from build123d import *

# Parameters (mm, degrees)
SKETCH1_R           = 2.55
SKETCH1_R_2         = 2.5
SKETCH1_R_3         = 10
BOSS_EXTRUDE1_DEPTH = 6.35


with BuildPart() as part:
    # Sketch1 → Boss-Extrude1 (new body)
    with BuildSketch(Plane(origin=(0, 0, 0), x_dir=(1, 0, 0), z_dir=(0, 1, 0))):
        with BuildLine():
            ThreePointArc((-155, 42.5), (-197.5, 0), (-155, -42.5))
            Line((-155, -42.5), (0, -42.5))
            ThreePointArc((0, -42.5), (42.200640469, -5.0354686), (10, 41.306779105))
            Line((10, 41.306779105), (10, 52.5))
            ThreePointArc((10, 52.5), (0, 62.5), (-10, 52.5))
            Line((-10, 52.5), (-10, 42.5))
            Line((-10, 42.5), (-155, 42.5))
        make_face()
        with BuildLine():
            ThreePointArc((-115, 2.55), (-112.45, 0), (-115, -2.55))
            Line((-115, -2.55), (-130, -2.55))
            ThreePointArc((-130, -2.55), (-132.55, 0), (-130, 2.55))
            Line((-130, 2.55), (-115, 2.55))
        make_face(mode=Mode.SUBTRACT)
        with Locations(Location((-155, -37.5, 0), (0, 0, 270))):
            Circle(SKETCH1_R, mode=Mode.SUBTRACT)
        with BuildLine():
            ThreePointArc((-155, -27.55), (-157.55, -25), (-155, -22.45))
            Line((-155, -22.45), (-140, -22.45))
            ThreePointArc((-140, -22.45), (-137.45, -25), (-140, -27.55))
            Line((-140, -27.55), (-155, -27.55))
        make_face(mode=Mode.SUBTRACT)
        with Locations(Location((-192.5, 0, 0), (0, 0, 270))):
            Circle(SKETCH1_R, mode=Mode.SUBTRACT)
        with BuildLine():
            ThreePointArc((-155, -10), (-165, 0), (-155, 10))
            Line((-155, 10), (-145, 10))
            ThreePointArc((-145, 10), (-135, 0), (-145, -10))
            Line((-145, -10), (-155, -10))
        make_face(mode=Mode.SUBTRACT)
        with BuildLine():
            ThreePointArc((-155, 22.45), (-157.55, 25), (-155, 27.55))
            Line((-155, 27.55), (-140, 27.55))
            ThreePointArc((-140, 27.55), (-137.45, 25), (-140, 22.45))
            Line((-140, 22.45), (-155, 22.45))
        make_face(mode=Mode.SUBTRACT)
        with Locations(Location((-155, 37.5, 0), (0, 0, 270))):
            Circle(SKETCH1_R, mode=Mode.SUBTRACT)
        with Locations(Location((0, 37.5, 0), (0, 0, 270))):
            Circle(SKETCH1_R, mode=Mode.SUBTRACT)
        with Locations(Location((17.67766953, 17.67766953, 0), (0, 0, 270))):
            Circle(SKETCH1_R_2, mode=Mode.SUBTRACT)
        with Locations(Location((-17.67766953, -17.67766953, 0), (0, 0, 270))):
            Circle(SKETCH1_R_2, mode=Mode.SUBTRACT)
        with Locations(Location((0, -37.5, 0), (0, 0, 270))):
            Circle(SKETCH1_R, mode=Mode.SUBTRACT)
        with Locations(Location((17.67766953, -17.67766953, 0), (0, 0, 270))):
            Circle(SKETCH1_R_2, mode=Mode.SUBTRACT)
        with Locations(Location((0, 0, 0), (0, 0, 270))):
            Circle(SKETCH1_R_3, mode=Mode.SUBTRACT)
        with Locations(Location((37.5, 0, 0), (0, 0, 270))):
            Circle(SKETCH1_R, mode=Mode.SUBTRACT)
        with Locations(Location((-17.67766953, 17.67766953, 0), (0, 0, 270))):
            Circle(SKETCH1_R_2, mode=Mode.SUBTRACT)
        with Locations(Location((0, 52.5, 0), (0, 0, 270))):
            Circle(SKETCH1_R_2, mode=Mode.SUBTRACT)
    extrude(amount=-BOSS_EXTRUDE1_DEPTH)


solid = part.part
Input: part model. Units: mm. Frame: model coordinates. A direction names the side the tool comes from. Give positions to 0.01 mm unless a question says otherwise; leave off trailing zeros. Loops run counter-clockwise (first coordinate to the right, second up) from the corner with the lowest first, then second, coordinate; pieces in that order, holes last. Notation, with made-up numbers: (82, -23) -> (101, -23) arc R21 ccw to (101, -17) -> close; hole circle Ø8 at (81, 11). An arc over 180 degrees is marked (long way). Answer as a JSON object with one key per item and string values. Group by question number.
Item 1: Pin query (flat end, axial travel): P1, Ø6.5, axis at x = -192.5, z = 0, coming from the +Y side; P2, Ø1, axis at x = 8, y = -5.5, coming from the -Z side; P3, Ø1.5, axis at y = -2.5, z = 4.5, coming from the -X side; P4, Ø1.9, axis at x = -147.5, y = -4, coming from the -Z side. Return the tip coordinate at first contact, or that it passes through.
Item 2: Reachability of faces 1 (the cylindrical face through (-157.55, -3.13, 25.06)), 2 (the flat face through (-10, -3, -48)), 3 (the flat face through (-79, 0, 1)) from +Z, -Z, +X, -X, +Y, -Y: full face, straight path, thin tool, end or side. Return the list, or none.
Item 3: Cut plane A-A, the plane z = -37.5. Return the cut outline in (x, y).
Item 4: Pull-direction query (Z, two-part tool) for faces 4 (the flat face through (10, -3, -47)), 5 (the cylindrical face through (-189.97, -3.13, -0.33)), 6 (the flat face through (-81, -3, -42.5)); classes: released by +Z, released by -Z, zero draft, split by the parting line, or undercut.
Item 5: Cut plane C-C, the plane x = -63. Return the cut outline in (y, z).
Item 6: Cut plane D-D, the plane y = -2.75. State how many separate pieces and enclosed holes the cut face has, and give its area (3 significant figures).
Item 7: Cut plane B-B, the plane z = -25. Return the cut outline in (x, y), and give its area (3 significant figures).
Item 8: Line query: probe 1 along X at (y, z) = (-2.25, 0); probe 2 along Z at (x, y) = (-153, -4); probe 3 along Z at (x, y) = (-118.5, -5.5). Output: solid intervals per line, ascending.
Checks:
{
 "1": {"P1": "stops at y = 0", "P2": "stops at z = -59.11", "P3": "stops at x = -197.33", "P4": "stops at z = -42.5"},
 "2": {"face 1": "+Y, -Y", "face 2": "-Z, -X, +Y, -Y", "face 3": "+Z, -Z, +X, -X, +Y"},
 "3": {"outline": "(-175, -6.35) -> (-157.55, -6.35) -> (-157.55, 0) -> (-175, 0) -> close; (-152.45, -6.35) -> (-2.55, -6.35) -> (-2.55, 0) -> (-152.45, 0) -> close; (2.55, -6.35) -> (20, -6.35) -> (20, 0) -> (2.55, 0) -> close"},
 "4": {"face 4": "zero draft", "face 5": "undercut", "face 6": "released by -Z"},
 "5": {"outline": "(-6.35, -42.5) -> (0, -42.5) -> (0, 42.5) -> (-6.35, 42.5) -> close"},
 "6": {"separate pieces": "1", "enclosed holes": "16", "area": "17,900 mm²"},
 "7": {"outline": "(-189.37, -6.35) -> (-157.55, -6.35) -> (-157.55, 0) -> (-189.37, 0) -> close; (-137.45, -6.35) -> (34.37, -6.35) -> (34.37, 0) -> (-137.45, 0) -> close", "area": "1,290 mm²"},
 "8": {"probe 1": "x = -197.5 to -195.05, -189.95 to -165, -135 to -132.55, -112.45 to -10, 10 to 34.95, 40.05 to 42.5", "probe 2": "z = -42.5 to -39.08, -35.92 to -27.55, -22.45 to -10, 10 to 22.45, 27.55 to 35.92, 39.08 to 42.5", "probe 3": "z = -42.5 to -2.55, 2.55 to 42.5"}
}
